from build123d import *

# Parameters (mm, degrees)
CROQUIS2_W              = 75
CROQUIS2_H              = 12.7
SALIENTE_EXTRUIR1_DEPTH = 6.35
CROQUIS3_R              = 2.3
CORTAR_EXTRUIR1_DEPTH   = 41.098160806


with BuildPart() as part:
    # Croquis2 → Saliente-Extruir1 (new, symmetric)
    with BuildSketch(Plane.XY):
        Rectangle(CROQUIS2_W, CROQUIS2_H)
        with BuildLine():
            ThreePointArc((0, 4.337049688), (-9.9, 0), (0, -4.337049688))
            ThreePointArc((0, -4.337049688), (9.9, 0), (0, 4.337049688))
        make_face(mode=Mode.SUBTRACT)
    extrude(amount=SALIENTE_EXTRUIR1_DEPTH, both=True)

    # Croquis3 → Cortar-Extruir1 (cut, through all)
    with BuildSketch(Plane(origin=(0, 6.35, 0), x_dir=(1, 0, 0), z_dir=(0, 1, 0))):
        with Locations(Location((32.5, 0, 0), (0, 0, 270))):
            Circle(CROQUIS3_R)
        with Locations(Location((22.5, 0, 0), (0, 0, 270))):
            Circle(CROQUIS3_R)
        with Locations(Location((-32.5, 0, 0), (0, 0, 90))):
            Circle(CROQUIS3_R)
        with Locations(Location((-22.5, 0, 0), (0, 0, 90))):
            Circle(CROQUIS3_R)
    extrude(amount=-CORTAR_EXTRUIR1_DEPTH, mode=Mode.SUBTRACT)


solid = part.part
Source: CAD feature listing. Evaluate the final solid. Frame: model axes, mm. Round coordinates to 2 decimals unless told otherwise and drop trailing zeros. Write each loop counter-clockwise with the first axis right and the second up, starting at its lowest first coordinate (ties: lowest second). Pieces come first, ordered by that corner, then holes. Notation, with made-up numbers: (83, 72) - (135, 72) arc R23 ccw to (135, 80) - close; hole circle Ø11 at (81.25, -5). An arc over 180 degrees is marked (long way). Use CSV: the item, a comma, the result in double quotes. Start each with the question number.
(1) Cut plane C-C, the plane z = -1. Return loops of the section in (x, y).
(2) Cut plane A-A, the plane x = 4. Return loops of the section in (y, z).
(3) First-contact query: pin 1 Ø4 at (x, y) = (0.5, 1) entering from +Z; pin 2 Ø6 at (x, z) = (22.5, 0) entering from -Y. Flat tips, straight axial feed; report the tip coordinate or a pass-through.
(4) Mould query, pull axis X, two halves, no side actions, for faces 1 (the face through (-1, 6.35, 0)), 2 (the face through (20.46, 0.09, 1.06)), 3 (the face through (37.5, 0, 0)). Classes: pulls with the +X half, pulls with the -X half, needs draft (parallel to the pull), parting line crosses it, or undercut.
(5) Material intervals for probe 1 along X at (y, z) = (0, 1); probe 2 along X at (y, z) = (3, -0.75); probe 3 along Z at (x, y) = (33.5, 4), sorted ascending. Write a range as [from, to].
(6) Cut plane B-B, the plane y = 0. Return loops of the section in (x, z).
(7) Cut plane D-D, the plane y = 3.5. Return loops of the section in (x, z).
Geometry says:
1,outline,"(-37.5, -6.35) - (-34.57, -6.35) - (-34.57, 6.35) - (-37.5, 6.35) - close; (-30.43, -6.35) - (-24.57, -6.35) - (-24.57, 6.35) - (-30.43, 6.35) - close; (-20.43, -6.35) - (20.43, -6.35) - (20.43, 6.35) - (-20.43, 6.35) - close; (24.57, -6.35) - (30.43, -6.35) - (30.43, 6.35) - (24.57, 6.35) - close; (34.57, -6.35) - (37.5, -6.35) - (37.5, 6.35) - (34.57, 6.35) - close; hole (0, -4.34) arc R5.9 ccw (long way) to (0, 4.34) arc R5.9 ccw (long way) to start"
2,outline,"(-6.35, -6.35) - (-5.9, -6.35) - (-5.9, 6.35) - (-6.35, 6.35) - close; (5.9, -6.35) - (6.35, -6.35) - (6.35, 6.35) - (5.9, 6.35) - close"
3,pin 1,"through"
3,pin 2,"y = -6.35"
4,face 1,"needs draft"
4,face 2,"undercut"
4,face 3,"pulls with the +X half"
5,probe 1,"[-37.5, -34.57], [-30.43, -24.57], [-20.43, -9.9], [9.9, 20.43], [24.57, 30.43], [34.57, 37.5]"
5,probe 2,"[-37.5, -34.67], [-30.33, -24.67], [-20.33, -9.08], [9.08, 20.33], [24.67, 30.33], [34.67, 37.5]"
5,probe 3,"[-6.35, -2.07], [2.07, 6.35]"
6,outline,"(-37.5, -6.35) - (-9.9, -6.35) - (-9.9, 6.35) - (-37.5, 6.35) - close; (9.9, -6.35) - (37.5, -6.35) - (37.5, 6.35) - (9.9, 6.35) - close; hole circle Ø4.6 at (-32.5, 0); hole circle Ø4.6 at (-22.5, 0); hole circle Ø4.6 at (22.5, 0); hole circle Ø4.6 at (32.5, 0)"
7,outline,"(-37.5, -6.35) - (-8.75, -6.35) - (-8.75, 6.35) - (-37.5, 6.35) - close; (8.75, -6.35) - (37.5, -6.35) - (37.5, 6.35) - (8.75, 6.35) - close; hole circle Ø4.6 at (-32.5, 0); hole circle Ø4.6 at (-22.5, 0); hole circle Ø4.6 at (22.5, 0); hole circle Ø4.6 at (32.5, 0)"
